CAD build for the part. Positions are in the model's coordinates, mm. Face numbers are marked on the shaded views. Give positions to 0.01 mm unless a question says otherwise; leave off trailing zeros. Loops run counter-clockwise (first coordinate to the right, second up) from the corner with the lowest first, then second, coordinate; pieces in that order, holes last. Notation, with made-up numbers: M 40.25,-18 L 94.25,-18 A27 ccw 94.25,2 Z; hole C 12,88 d3. An arc over 180 degrees is marked long. Answer as CSV lines item,"result".
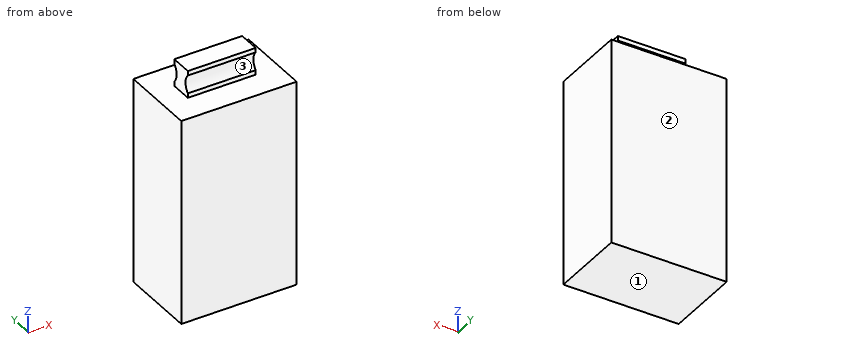
```python
from build123d import *

# Parameters (mm, degrees)
SKETCH1_W           = 51
SKETCH1_H           = 34
BOSS_EXTRUDE1_DEPTH = 91
SKETCH2_W           = 30
SKETCH2_H           = 6
BOSS_EXTRUDE2_DEPTH = 12
BOSS_EXTRUDE3_DEPTH = 30


with BuildPart() as part:
    # Sketch1 → Boss-Extrude1 (new body)
    with BuildSketch(Plane.XY):
        with Locations((25.5, -17)):
            Rectangle(SKETCH1_W, SKETCH1_H)
    extrude(amount=BOSS_EXTRUDE1_DEPTH)

    # Sketch2 → Boss-Extrude2 (add)
    with BuildSketch(Plane.XY.offset(91)):
        with Locations((25.5, -17)):
            Rectangle(SKETCH2_W, SKETCH2_H)
    extrude(amount=BOSS_EXTRUDE2_DEPTH)

    # Sketch3 → Boss-Extrude3 (add)
    with BuildSketch(Plane.ZY.offset(-10.5)):
        with BuildLine():
            Line((91, -12.2), (93, -12.2))
            ThreePointArc((93, -12.2), (97, -13.856854249), (101, -12.2))
            Line((101, -12.2), (103, -12.2))
            Line((103, -12.2), (103, -14))
            Line((103, -14), (91, -14))
            Line((91, -14), (91, -12.2))
        make_face()
        with BuildLine():
            Line((103, -20), (103, -21.8))
            Line((103, -21.8), (101, -21.8))
            ThreePointArc((101, -21.8), (97, -20.143145751), (93, -21.8))
            Line((93, -21.8), (91, -21.8))
            Line((91, -21.8), (91, -20))
            Line((91, -20), (103, -20))
        make_face()
    extrude(amount=-BOSS_EXTRUDE3_DEPTH)


solid = part.part
```
Q1. Cut at B-B (y = -7.5). Write the cut outline in (x, z), and give its area (3 significant figures).
Solution:
outline,"M 0,0 L 51,0 L 51,91 L 0,91 Z"
area,"4,640 mm²"
Q2. Cut at A-A (x = 13.5). Write the cut outline in (y, z).
Solution:
outline,"M -34,0 L 0,0 L 0,91 L -12.2,91 L -12.2,93 A5.66 cw -12.2,101 L -12.2,103 L -21.8,103 L -21.8,101 A5.66 cw -21.8,93 L -21.8,91 L -34,91 Z"
Q3. Pin check, flat tips, straight feed: P1, Ø0.6, axis at x = 31.5, z = 102.5, coming from the -Y side; P2, Ø2, axis at x = 26.5, z = 102, coming from the +Y side; P3, Ø10.5, axis at y = -17, z = 99.5, coming from the -X side. Stop position of each tip, or through.
Solution:
P1,"stops at y = -21.8"
P2,"stops at y = -12.2"
P3,"stops at x = 10.5"
Q4. Wall check: line 1 (Z direction, x = 21, y = -23). Give the ranges that are in metal, low to high. Write a range as [from, to].
Solution:
line 1,"z = [0, 91]"
Q5. Mould opens along Z. For the marked faces 1, 2 and 3 say: released by +Z, released by -Z, zero draft, split by the parting line, or undercut.
Solution:
face 1,"released by -Z"
face 2,"zero draft"
face 3,"undercut"
